Model file for the job. Use its own axes, mm. A direction names the side the tool comes from. Round coordinates to 2 decimals unless told otherwise and drop trailing zeros. Order: outer loops, then holes, each group sorted by start corner. A loop starts at its lowest first (then second) coordinate and runs counter-clockwise, first axis right, second up. Notation, with made-up numbers: M -6.5,51 L 11.5,51 A15 ccw 11.5,79 Z; hole C 6,46 d5. An arc over 180 degrees is marked long. Return JSON: item names as keys, results as strings. Group by question number.
Item 1: Slice it at C-C on x = 0.5. Write the cut outline in (y, z), then the cut area to 3 significant figures.
Item 2: Probe line 1 along Z through (x, y) = (28.5, 15.5); line 2 along Z through (x, y) = (-6.5, 34); line 3 along Y through (x, z) = (57, 12). List the from-to ranges inside material, lowest first.
Item 3: Pull direction Z, two halves, no side cores. Call faces 1 (the face through (-1, 17, -29)), 2 (the face through (-45, 14, 0)), 3 (the face through (-1, 38, -22)): pulls with the +Z half, pulls with the -Z half, needs draft (parallel to the pull), parting line crosses it, or undercut.
Item 4: Slice it at A-A on z = 0. Write the cut outline in (x, y).
Item 5: Slice it at B-B on x = -33. Write the cut outline in (y, z), then the cut area to 3 significant figures.
Item 6: Which spindle directions (+Z, -Z, +X, -X, +Y, -Y) get a long thin tool onto all of the face, cutting with end or side? Do faces 4 (the face through (1, 33, -18)), 5 (the face through (-1, 38, 22)), 6 (the face through (-52.5, 6, 0)), 7 (the face through (13, 14, 0)), 8 (the face through (52.5, 6, 0)). Say none if no direction does.
Item 7: Slice it at D-D on z = 24. Write the cut outline in (x, y).
Item 8: Pin check, flat tips, straight feed: pin 1 Ø1.5 at (y, z) = (20.5, 14.5) entering from -X; pin 2 Ø6.5 at (y, z) = (8.5, 13) entering from -X; pin 3 Ø4 at (x, z) = (10, 8.5) entering from +Y. Stop position of each tip, or through.
from build123d import *

# Parameters (mm, degrees)
ESQUISSE1_W                 = 127
ESQUISSE1_H                 = 58
CREATION_PREMIER_CUBE_DEPTH = 38
ESQUISSE2_W                 = 11
ESQUISSE2_H                 = 58
ENLEVE_RECLANGLE_BAS_DEPTH  = 13
CONG_15_START               = -30
CONG_15_DEPTH               = 60
CONG_16_START               = -30
CONG_16_DEPTH               = 60
ENL_V_MAT_EXTRU_7_DEPTH     = 11
ENL_V_MAT_EXTRU_10_DEPTH    = 50
ENL_V_MAT_EXTRU_11_DEPTH    = 50
CONG_18_R                   = 3


with BuildPart() as part:
    # Esquisse1 → Creation premier cube (new body)
    with BuildSketch(Plane(origin=(0, 0, 0), x_dir=(1, 0, 0), z_dir=(0, 1, 0))):
        Rectangle(ESQUISSE1_W, ESQUISSE1_H)
    extrude(amount=CREATION_PREMIER_CUBE_DEPTH)

    # Esquisse2 → Enleve reclangle bas (cut)
    with BuildSketch(Plane.XZ):
        with Locations((58, 0)):
            Rectangle(ESQUISSE2_W, ESQUISSE2_H)
        with Locations((-58, 0)):
            Rectangle(ESQUISSE2_W, ESQUISSE2_H)
    extrude(amount=-ENLEVE_RECLANGLE_BAS_DEPTH, mode=Mode.SUBTRACT)

    # Congé15: read off the stored shape, not the designer's step
    # Congé15 outline → Congé15 (cut)
    with BuildSketch(Plane.XY.offset(CONG_15_START)):
        with BuildLine():
            Line((-63.5, 38), (-63.5, 17.493903346))
            ThreePointArc((-63.5, 17.493903346), (-57.493903346, 31.993903346), (-42.993903346, 38))
            Line((-42.993903346, 38), (-63.5, 38))
        make_face()
    extrude(amount=CONG_15_DEPTH, mode=Mode.SUBTRACT)

    # Congé16: read off the stored shape, not the designer's step
    # Congé16 outline → Congé16 (cut)
    with BuildSketch(Plane.XY.offset(CONG_16_START)):
        with BuildLine():
            ThreePointArc((42.993903346, 38), (57.493903346, 31.993903346), (63.5, 17.493903346))
            Line((63.5, 17.493903346), (63.5, 38))
            Line((63.5, 38), (42.993903346, 38))
        make_face()
    extrude(amount=CONG_16_DEPTH, mode=Mode.SUBTRACT)

    # Esquisse9 → Enlèv. mat.-Extru.7 (cut)
    with BuildSketch(Plane(origin=(0, 38, 0), x_dir=(1, 0, 0), z_dir=(0, 1, 0))):
        Polygon((-0.380283646, 18), (-63.5, 18), (-63.5, -18), (-0.380283646, -18), (63.5, -18), (63.5, 18), align=None)
    extrude(amount=-ENL_V_MAT_EXTRU_7_DEPTH, mode=Mode.SUBTRACT)

    # Esquisse10 → Enlèv. mat.-Extru.10 (cut)
    with BuildSketch(Plane(origin=(0, 27, 0), x_dir=(1, 0, 0), z_dir=(0, 1, 0))):
        with BuildLine():
            Line((-38.5, -6.5), (-19.5, -6.5))
            ThreePointArc((-19.5, -6.5), (-13, 0), (-19.5, 6.5))
            Line((-19.5, 6.5), (-38.5, 6.5))
            ThreePointArc((-38.5, 6.5), (-45, 0), (-38.5, -6.5))
        make_face()
    extrude(amount=-ENL_V_MAT_EXTRU_10_DEPTH, mode=Mode.SUBTRACT)

    # Esquisse10<3> → Enlèv. mat.-Extru.11 (cut)
    with BuildSketch(Plane(origin=(0, 27, 0), x_dir=(1, 0, 0), z_dir=(0, 1, 0))):
        with BuildLine():
            Line((38.5, -6.5), (19.5, -6.5))
            ThreePointArc((19.5, -6.5), (13, 0), (19.5, 6.5))
            Line((19.5, 6.5), (38.5, 6.5))
            ThreePointArc((38.5, 6.5), (45, 0), (38.5, -6.5))
        make_face()
        with BuildLine():
            Line((-38.5, -6.5), (-19.5, -6.5))
            ThreePointArc((-19.5, -6.5), (-13, 0), (-19.5, 6.5))
            Line((-19.5, 6.5), (-38.5, 6.5))
            ThreePointArc((-38.5, 6.5), (-45, 0), (-38.5, -6.5))
        make_face()
    extrude(amount=-ENL_V_MAT_EXTRU_11_DEPTH, mode=Mode.SUBTRACT)

    # Congé18
    cong_18_edges = [part.edges().sort_by_distance(p)[0] for p in [
        (-63.5, 15.246951673, -29),
        (-63.5, 15.246951673, 29),
        (0, 38, 29),
        (-57.493903346, 31.993903346, 29),
        (-57.493903346, 31.993903346, -29),
        (63.5, 15.246951673, -29),
        (63.5, 15.246951673, 29),
        (0, 38, -29),
        (57.493903346, 31.993903346, -29),
        (57.493903346, 31.993903346, 29),
    ]]
    fillet(cong_18_edges, radius=CONG_18_R)


solid = part.part
Output values:
{
 "1": {"outline": "M 0,-29 L 35,-29 A3 ccw 38,-26 L 38,-18 L 27,-18 L 27,18 L 38,18 L 38,26 A3 ccw 35,29 L 0,29 Z", "area": "1,800 mm²"},
 "2": {"line 1": "-29 to -6.5, 6.5 to 29", "line 2": "-29 to -18, 18 to 29", "line 3": "13 to 27"},
 "3": {"face 1": "pulls with the -Z half", "face 2": "undercut", "face 3": "needs draft"},
 "4": {"outline": "M -63.5,13 L -52.5,13 L -52.5,0 L -45,0 L -45,27 L -61.16,27 A20.51 ccw -63.5,17.49 Z; M -13,0 L 13,0 L 13,27 L -13,27 Z; M 45,0 L 52.5,0 L 52.5,13 L 63.5,13 L 63.5,17.49 A20.51 ccw 61.16,27 L 45,27 Z"},
 "5": {"outline": "M 0,-29 L 35,-29 A3 ccw 38,-26 L 38,-18 L 27,-18 L 27,-6.5 L 0,-6.5 Z; M 0,6.5 L 27,6.5 L 27,18 L 38,18 L 38,26 A3 ccw 35,29 L 0,29 Z", "area": "1,450 mm²"},
 "6": {"face 4": "+X, -X, +Y", "face 5": "+Z, -Z, +X, -X, +Y", "face 6": "+Z, -Z, -X, -Y", "face 7": "+Y, -Y", "face 8": "+Z, -Z, +X, -Y"},
 "7": {"outline": "M -63.5,13 L -52.5,13 L -52.5,0 L 52.5,0 L 52.5,13 L 63.5,13 L 63.5,17.49 A20.51 ccw 42.99,38 L -42.99,38 A20.51 ccw -63.5,17.49 Z"},
 "8": {"pin 1": "x = -63.38", "pin 2": "x = -52.5", "pin 3": "y = 27"}
}
